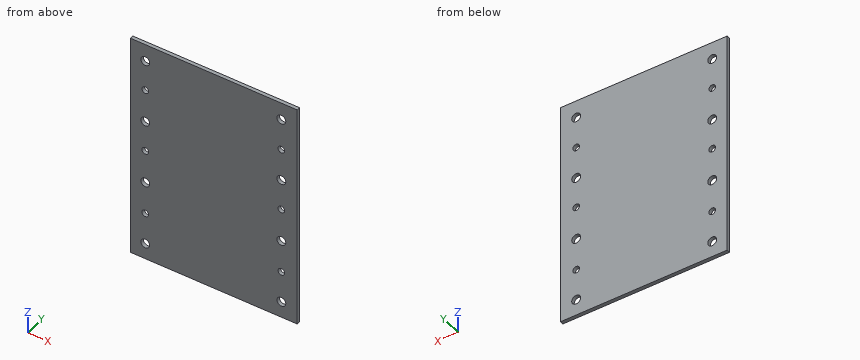
Autodesk Inventor part; units mm, degrees
ref_plane "YZ Plane" through (0, 0, 0) normal (1, 0, 0) x (0, 1, 0)
ref_plane "XZ Plane" through (0, 0, 0) normal (0, 1, 0) x (-1, 0, 0)
ref_plane "XY Plane" through (0, 0, 0) normal (0, 0, 1) x (1, 0, 0)
sketch "Sketch1" plane through (0, 0, 0) normal (0, 1, 0) x (-1, 0, 0)
  line L0 (0, 0) -> (75, 0)
  line L1 (75, 0) -> (75, -100)
  line L2 (75, -100) -> (0, -100)
  line L3 (0, -100) -> (0, 0)
  circle A0 centre (68.28, -7.71) radius 2
  circle A1 centre (68.28, -35.95) radius 2
  circle A2 centre (68.28, -64.35) radius 2
  circle A3 centre (68.28, -92.9) radius 2
  circle A4 centre (7.12, -7.71) radius 2
  circle A5 centre (7.12, -35.95) radius 2
  circle A6 centre (7.12, -64.4) radius 2
  circle A7 centre (7.12, -92.8) radius 2
  circle A8 centre (7.12, -21.73) radius 1.5
  circle A9 centre (7.12, -49.67) radius 1.5
  circle A10 centre (7.12, -78.83) radius 1.5
  circle A11 centre (68.28, -21.28) radius 1.5
  circle A12 centre (68.28, -49.62) radius 1.5
  circle A13 centre (68.28, -78.83) radius 1.5
  line L4 (68.28, 0) -> (68.28, -100) construction
  line L5 (7.12, 0) -> (7.12, -100) construction
  dimension "d0" = 75
  dimension "d1" = 100
  dimension "d2" = 7.12
  dimension "d3" = 6.72
  dimension "d4" = 4
  dimension "d5" = 3
  dimension "d6" = 4
  dimension "d7" = 3
  dimension "d8" = 4
  dimension "d9" = 3
  dimension "d10" = 4
  dimension "d11" = 4
  dimension "d12" = 3
  dimension "d13" = 4
  dimension "d14" = 3
  dimension "d15" = 4
  dimension "d16" = 3
  dimension "d17" = 4
  dimension "d18" = 7.71
  dimension "d19" = 21.73
  dimension "d20" = 35.95
  dimension "d21" = 49.67
  dimension "d22" = 64.4
  dimension "d23" = 78.83
  dimension "d24" = 92.8
  dimension "d25" = 7.71
  dimension "d26" = 21.28
  dimension "d27" = 35.95
  dimension "d28" = 49.62
  dimension "d29" = 64.35
  dimension "d30" = 78.83
  dimension "d31" = 92.9
extrude "Extrusion1" add sketch "Sketch1" along normal blind 1.6
properties part number "Placa"
Source: CAD feature listing. Evaluate the final solid. Frame: model axes, mm. Give positions to 0.01 mm unless a question says otherwise; leave off trailing zeros. Write each loop counter-clockwise with the first axis right and the second up, starting at its lowest first coordinate (ties: lowest second). Pieces come first, ordered by that corner, then holes. Notation, with made-up numbers: (15, -16.5) - (20, -16.5) arc R16 cw to (20, -12.5) - close; hole circle Ø11 at (7.5, 74). An arc over 180 degrees is marked (long way). Write item = value, one per line. Start each with the question number.
Q1. Cut plane B-B, the plane z = -7.71. Return loops of the section in (x, y).
Q2. Pin query (flat end, axial travel): pin 1 Ø6.5 at (x, z) = (-68.28, -64.35) entering from +Y. Return the tip coordinate at first contact, or that it passes through.
Q3. Cut plane A-A, the plane x = -68.28. Give the number of separate pieces and of enclosed holes in the cut face, then the cut area to 3 significant figures.
Q4. Material intervals for probe 1 along X at (y, z) = (0.6, -49.5); probe 2 along X at (y, z) = (0.9, -92), sorted ascending.
Q5. Cut plane D-D, the plane z = -78.83. Return loops of the section in (x, y).
Computed values:
q1.outline = (-75, 0) - (-70.28, 0) - (-70.28, 1.6) - (-75, 1.6) - close; (-66.28, 0) - (-9.12, 0) - (-9.12, 1.6) - (-66.28, 1.6) - close; (-5.12, 0) - (0, 0) - (0, 1.6) - (-5.12, 1.6) - close
q2.pin_1 = 1.6
q3.separate_pieces = 8
q3.enclosed_holes = 0
q3.area = 120 mm²
q4.probe_1 = -75 to -69.78, -66.78 to -8.61, -5.63 to 0
q4.probe_2 = -75 to -70.07, -66.49 to -8.95, -5.29 to 0
q5.outline = (-75, 0) - (-69.78, 0) - (-69.78, 1.6) - (-75, 1.6) - close; (-66.78, 0) - (-8.62, 0) - (-8.62, 1.6) - (-66.78, 1.6) - close; (-5.62, 0) - (0, 0) - (0, 1.6) - (-5.62, 1.6) - close
